Source: three-view drawing plus pictorial views. Frame: mm from the lowest corner of the part. A direction names the side the tool comes from. Coordinates: 2 decimals unless noted, no trailing zeros. Loops run counter-clockwise (first coordinate to the right, second up) from the corner with the lowest first, then second, coordinate; pieces in that order, holes last. Notation, with made-up numbers: (77.5, 23.5) - (129.5, 23.5) arc R23 cw to (129.5, 62.5) - close; hole circle Ø11 at (48.25, 80.5). An arc over 180 degrees is marked (long way). Return JSON: item names as keys, results as strings.
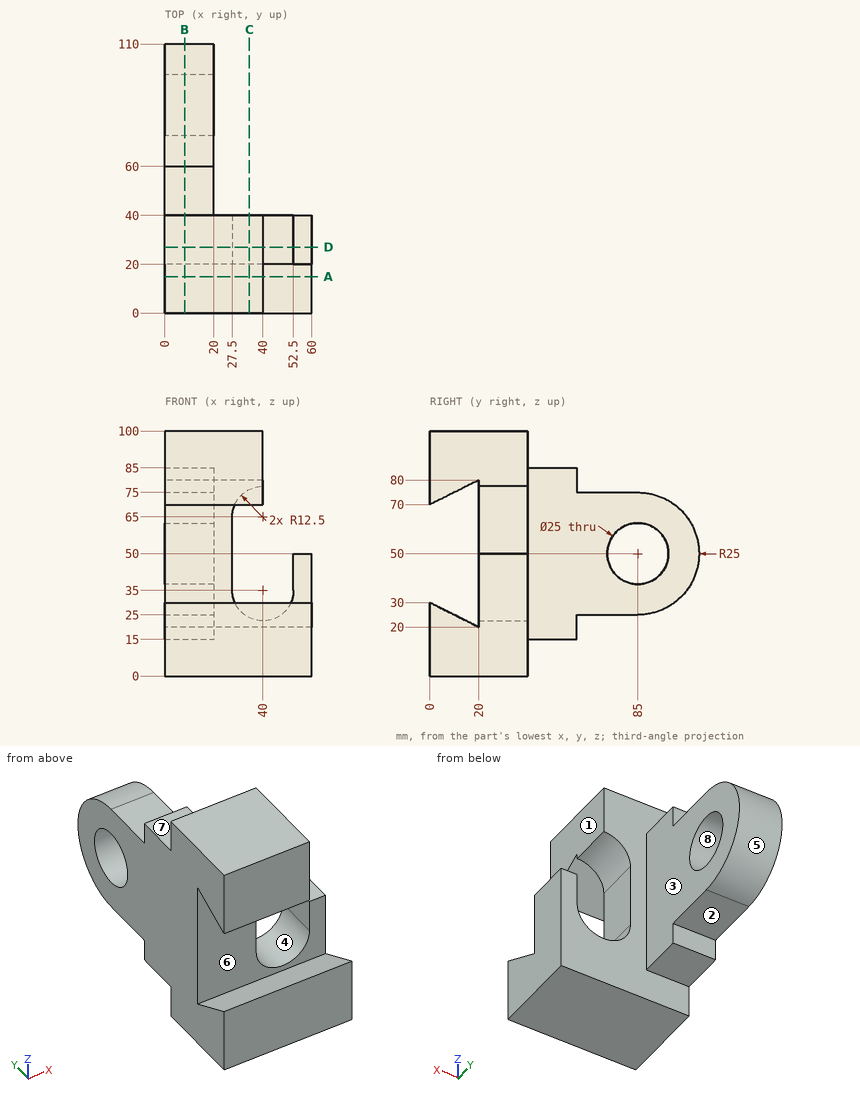
Item 1: Mould query, pull axis Y, two halves, no side actions, for the marked faces 5, 6, 7 and 8. Classes: +Y half, -Y half, draft (parallel to the pull), parting line (faces both ways), or undercut.
Worked out:
{"face 5": "+Y half", "face 6": "undercut", "face 7": "draft", "face 8": "undercut"}
Item 2: First-contact query: pin 1 Ø6 at (x, z) = (19.5, 72.5) entering from +Y; pin 2 Ø6 at (x, y) = (10.5, 46) entering from -Z; pin 3 Ø24 at (y, z) = (22, 91) entering from +X. Flat tips, straight axial feed; report the tip coordinate or a pass-through.
Worked out:
{"pin 1": "y = 100.64", "pin 2": "z = 15", "pin 3": "x = 40"}
Item 3: Section query B-B, the plane x = 8. Return loops of the section in (y, z).
Worked out:
{"outline": "(0, 0) - (40, 0) - (40, 15) - (60, 15) - (60, 25) - (85, 25) arc R25 ccw to (85, 75) - (60, 75) - (60, 85) - (40, 85) - (40, 100) - (0, 100) - (0, 70) - (20, 80) - (20, 20) - (0, 30) - close; hole circle Ø25 at (85, 50)"}
Item 4: Ray query, probe 1 along Y at (x, z) = (5, 50); probe 2 along X at (y, z) = (8, 95); probe 3 along Z at (x, y) = (35.5, 28). Return the intervals inside material, ascending. Write a range as from..to.
Worked out:
{"probe 1": "20..72.5, 97.5..110", "probe 2": "0..40", "probe 3": "0..23.34, 76.66..100"}
Item 5: Section query C-C, the plane x = 34.5. Return loops of the section in (y, z), and give its area (3 significant figures).
Worked out:
{"outline": "(0, 0) - (40, 0) - (40, 23.78) - (20, 23.78) - (20, 20) - (0, 30) - close; (0, 70) - (20, 80) - (20, 76.22) - (40, 76.22) - (40, 100) - (0, 100) - close", "area": "1,950 mm^2"}
Item 6: Section query D-D, the plane y = 27. Return loops of the section in (x, z), and give its area (3 significant figures).
Worked out:
{"outline": "(0, 0) - (60, 0) - (60, 50) - (52.5, 50) - (52.5, 35) arc R12.5 cw to (27.5, 35) - (27.5, 65) arc R12.5 cw to (40, 77.5) - (40, 100) - (0, 100) - close", "area": "4,070 mm^2"}
Item 7: Reachability of the marked faces 1, 2, 3 and 4 from +Z, -Z, +X, -X, +Y, -Y: full face, straight path, thin tool, end or side. Return the list, or none.
Worked out:
{"face 1": "+Z, +X, +Y, -Y", "face 2": "-Z, +X, -X, +Y", "face 3": "+Z, -Z, +X, +Y", "face 4": "+Y"}
Item 8: Section query A-A, the plane y = 15. Return loops of the section in (x, z), and give its area (3 significant figures).
Worked out:
{"outline": "(0, 0) - (60, 0) - (60, 22.5) - (0, 22.5) - close; (0, 77.5) - (40, 77.5) - (40, 100) - (0, 100) - close", "area": "2,250 mm^2"}
